The listing builds one solid part. Answer for the finished solid, in the listing's coordinates (mm). A direction names the side the tool comes from. Give positions to 0.01 mm unless a question says otherwise; leave off trailing zeros. Order: outer loops, then holes, each group sorted by start corner. A loop starts at its lowest first (then second) coordinate and runs counter-clockwise, first axis right, second up.
```python
from build123d import *

# Parameters (mm, degrees)
BOSS_EXTRUDE1_DEPTH = 2.54
SKETCH2_OUTSIDE_W   = 31.388
SKETCH2_OUTSIDE_H   = 32.764
SKETCH2_OUTSIDE_R   = 4.445
CUT_EXTRUDE1_DEPTH  = 5.08
CUT_EXTRUDE1_DRAFT  = -60
SKETCH3_R           = 3.302
BOSS_EXTRUDE2_DEPTH = 76.2


with BuildPart() as part:
    # Sketch1 → Boss-Extrude1 (new, symmetric)
    with BuildSketch(Plane(origin=(0, 0, 0), x_dir=(1, 0, 0), z_dir=(0, 1, 0))):
        Polygon((0, 5.132643893), (-4.445, 2.566321947), (-4.445, -2.566321947), (0, -5.132643893), (4.445, -2.566321947), (4.445, 2.566321947), align=None)
    extrude(amount=BOSS_EXTRUDE1_DEPTH, both=True)


with BuildPart() as cut_extrude1_tool:
    # Sketch2 outside → Cut-Extrude1 (with draft: the straight prism first)
    with BuildSketch(Plane(origin=(0, 2.54, 0), x_dir=(1, 0, 0), z_dir=(0, 1, 0))):
        Rectangle(SKETCH2_OUTSIDE_W, SKETCH2_OUTSIDE_H)
        Circle(SKETCH2_OUTSIDE_R, mode=Mode.SUBTRACT)
    extrude(amount=-CUT_EXTRUDE1_DEPTH)
    # Cut-Extrude1: the draft: its side faces are tilted about the plane it starts from
    cut_extrude1_sides = [cut_extrude1_tool.faces().sort_by_distance(p)[0] for p in [
        (0, 0, 16.382),
        (15.694, 0, 0),
        (0, 0, -16.382),
        (-15.694, 0, 0),
        (-4.445, 0, 0),
    ]]
    draft(cut_extrude1_sides, Plane(origin=(0, 2.54, 0), x_dir=(1, 0, 0), z_dir=(0, 1, 0)), CUT_EXTRUDE1_DRAFT)


with BuildPart() as part_1:
    add(part.part)

    # Cut-Extrude1: cut by cut_extrude1_tool
    add(cut_extrude1_tool.part, mode=Mode.SUBTRACT)

    # Sketch3 → Boss-Extrude2 (add)
    with BuildSketch(Plane(origin=(0, -2.54, 0), x_dir=(-1, 0, 0), z_dir=(0, -1, 0))):
        with Locations(Location((0, 0, 0), (0, 0, 270))):
            Circle(SKETCH3_R)
    extrude(amount=BOSS_EXTRUDE2_DEPTH)


solid = part_1.part
```
1) Straight lines are drawn through the part: probe 1 along Y at (x, z) = (-1.25, 3.25); probe 2 along X at (y, z) = (-49, 0.25). For each, find the intervals that lie inside material, in ascending order.
Geometry says:
probe 1: y = -2.54 to 2.54
probe 2: x = -3.29 to 3.29
2) A tool of negligible diameter and unlimited length cuts with its end or side. For faces 1 (the cylindrical face through (-0.99, -40.11, 3.15)), 2 (the conical face through (3.986, 2.445, 2.314)), from which of +Z, -Z, +X, -X, +Y, -Y can it reach the whole face along a straight path? Write none if from no direction.
Geometry says:
face 1: -Y
face 2: +Z, +X, +Y
3) Given P1, Ø4, axis at x = 0.5, y = -42.5, coming from the -Z side; P2, Ø2, axis at x = -2.5, z = -4, coming from the -Y side; P3, Ø3, axis at y = -46, z = 1, coming from the -X side, each flat-ended and moving along its own axis, determine where each tip first touches the part or whether it passes through.
Geometry says:
P1: stops at z = -3.3
P2: stops at y = -2.54
P3: stops at x = -3.3
4) Find section A-A (y = -37.5). Write down the section's boundary in (x, z).
Geometry says:
outline: circle Ø6.6 at (0, 0)
